Study the drawing (mm; zero at the part's minimum x, y, z) and answer. Give positions to 0.01 mm unless a question says otherwise; leave off trailing zeros. Order: outer loops, then holes, each group sorted by start corner. A loop starts at its lowest first (then second) coordinate and runs counter-clockwise, first axis right, second up. Notation, with made-up numbers: (42.5, 88) - (76.5, 88) arc R30 ccw to (76.5, 115) - close; hole circle Ø3 at (44, -33). An arc over 180 degrees is marked (long way). Return JSON: item names as keys, results as strings.
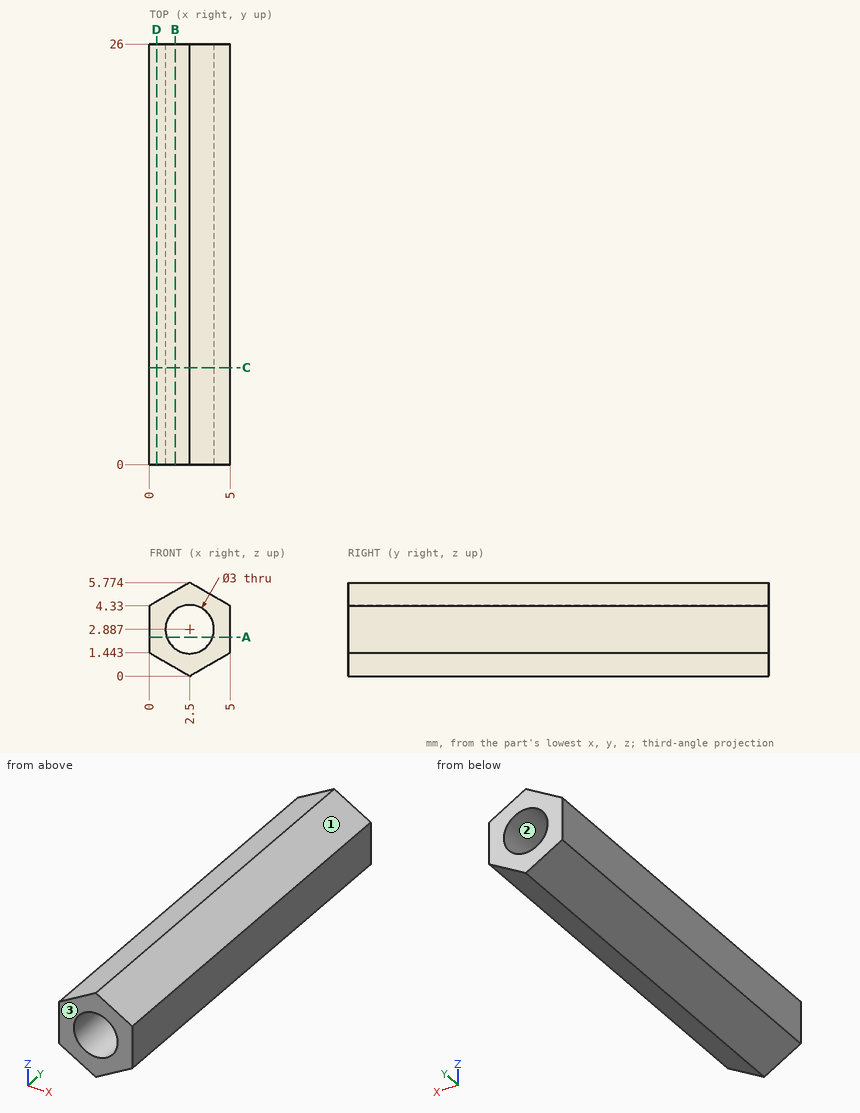
Q1. A cutting plane is placed at C-C (y = 6). Write down the section's boundary in (x, z).
Values:
{"outline": "(0, 1.44) - (2.5, 0) - (5, 1.44) - (5, 4.33) - (2.5, 5.77) - (0, 4.33) - close; hole circle Ø3 at (2.5, 2.89)"}
Q2. Consider L1, parallel to X at y = 17, z = 3 (1 decimal); L2, parallel to Z at x = 2.65, y = 23 (1 decimal); L3, parallel to Z at x = 1.45, y = 1.5 (1 decimal). Determine where each line is inside the solid, lowest interval first.
Values:
{"L1": "x = 0 to 1, 4 to 5", "L2": "z = 0.1 to 1.4, 4.4 to 5.7", "L3": "z = 0.6 to 1.8, 4 to 5.2"}
Q3. Determine the mould class of the marked faces 1, 2 and 3 for opening direction X: released by +X, released by -X, zero draft, split by the parting line, or undercut.
Values:
{"face 1": "released by +X", "face 2": "undercut", "face 3": "zero draft"}
Q4. A cutting plane is placed at A-A (z = 2.4). Write down the section's boundary in (x, y).
Values:
{"outline": "(0, 0) - (1.08, 0) - (1.08, 26) - (0, 26) - close; (3.92, 0) - (5, 0) - (5, 26) - (3.92, 26) - close"}
Q5. A cutting plane is placed at D-D (x = 0.45). Write down the section's boundary in (y, z).
Values:
{"outline": "(0, 1.18) - (26, 1.18) - (26, 4.59) - (0, 4.59) - close"}
Q6. A cutting plane is placed at B-B (x = 1.6). Write down the section's boundary in (y, z).
Values:
{"outline": "(0, 0.52) - (26, 0.52) - (26, 1.69) - (0, 1.69) - close; (0, 4.09) - (26, 4.09) - (26, 5.25) - (0, 5.25) - close"}
